For this review, take the finished solid that the model builds, in its own axes (mm). Face numbers are marked on the shaded views. A direction names the side the tool comes from. Round coordinates to 2 decimals unless told otherwise and drop trailing zeros. Order: outer loops, then holes, each group sorted by start corner. A loop starts at its lowest first (then second) coordinate and runs counter-clockwise, first axis right, second up. Notation, with made-up numbers: M 53,56.5 L 76,56.5 A8 cw 76,63.5 Z; hole C -31.5,80.5 d9. An arc over 180 degrees is marked long. Answer in a Markdown table with one row per item. Add a question column.
```python
from build123d import *

# Parameters (mm, degrees)
SKETCH1_R           = 0.499999685
SKETCH1_R_2         = 0.499999936
SKETCH1_R_3         = 3.000000209
SKETCH1_R_4         = 0.750000452
SKETCH1_R_5         = 0.748506913
SKETCH1_R_6         = 1.500187581
BOSS_EXTRUDE1_DEPTH = 4


# Read off the part's stored shape, not the designer's step: Imported1
with BuildPart() as part:
    # Sketch1 → Boss-Extrude1 (new body)
    with BuildSketch(Plane(origin=(0, 0, 0), x_dir=(-1, 0, 0), z_dir=(0, 0, -1))):
        with BuildLine():
            ThreePointArc((-10.3249643, 42.429967422), (-13.429964129, 45.534967549), (-16.534963959, 42.429967422))
            Line((-16.534963959, 42.429967422), (-16.534963959, 22.759328173))
            ThreePointArc((-16.534963959, 22.759328173), (-22.936546798, 10.91939696), (-11.523821193, 3.783997304))
            Line((-11.523821193, 3.783997304), (-11.151510993, 1.898050354))
            ThreePointArc((-11.151510993, 1.898050354), (-7.958448418, 0.172164331), (-6.866399752, 3.633632355))
            Line((-6.866399752, 3.633632355), (-6.907151039, 3.694454964))
            Line((-6.907151039, 3.694454964), (-7.95702579, 5.261426867))
            ThreePointArc((-7.95702579, 5.261426867), (-8.261161621, 6.315782715), (-7.802888126, 7.312853556))
            Line((-7.802888126, 7.312853556), (-7.336401059, 7.778170532))
            ThreePointArc((-7.336401059, 7.778170532), (-6.328947455, 8.250313315), (-5.25191043, 7.971256294))
            Line((-5.25191043, 7.971256294), (-3.681946925, 6.898545358))
            ThreePointArc((-3.681946925, 6.898545358), (-0.18308636, 7.931946592), (-1.898741108, 11.151647221))
            Line((-1.898741108, 11.151647221), (-3.784109013, 11.52325713))
            ThreePointArc((-3.784109013, 11.52325713), (-4.744145314, 12.052872295), (-5.125871494, 13.080708395))
            Line((-5.125871494, 13.080708395), (-5.125914366, 13.778599746))
            Line((-5.125914366, 13.778599746), (-5.125914378, 13.778793202))
            ThreePointArc((-5.125914378, 13.778793202), (-4.744155373, 14.806645767), (-3.783994211, 15.336090171))
            Line((-3.783994211, 15.336090171), (-1.90356186, 15.70732102))
            ThreePointArc((-1.90356186, 15.70732102), (-0.193583134, 18.935202355), (-3.703637126, 19.946521356))
            Line((-3.703637126, 19.946521356), (-5.261386695, 18.902842274))
            ThreePointArc((-5.261386695, 18.902842274), (-6.314757765, 18.59870429), (-7.311417899, 19.055605922))
            Line((-7.311417899, 19.055605922), (-7.805450119, 19.549549653))
            ThreePointArc((-7.805450119, 19.549549653), (-8.262234293, 20.54598288), (-7.957754629, 21.598989571))
            Line((-7.957754629, 21.598989571), (-6.908352, 23.163741071))
            Line((-6.908352, 23.163741071), (-6.866399752, 23.226295558))
            ThreePointArc((-6.866399752, 23.226295558), (-6.774111326, 25.630427698), (-8.842129144, 26.859927922))
            Line((-8.842129144, 26.859927922), (-10.3249643, 26.859927922))
            Line((-10.3249643, 26.859927922), (-10.3249643, 42.429967422))
        make_face()
        with Locations(Location((-15.179963978, 6.929964102, 0), (0, 0, 90))):
            Circle(SKETCH1_R, mode=Mode.SUBTRACT)
        with Locations(Location((-11.679964298, 6.929964382, 0), (0, 0, 90))):
            Circle(SKETCH1_R_2, mode=Mode.SUBTRACT)
        with Locations(Location((-13.42996461, 13.429962781, 0), (0, 0, 90))):
            Circle(SKETCH1_R_3, mode=Mode.SUBTRACT)
        with Locations(Location((-15.179964076, 20.429963954, 0), (0, 0, 90))):
            Circle(SKETCH1_R_4, mode=Mode.SUBTRACT)
        with Locations(Location((-11.681540167, 20.429629577, 0), (0, 0, 90))):
            Circle(SKETCH1_R_5, mode=Mode.SUBTRACT)
        with Locations(Location((-13.429420254, 42.425723706, 0), (0, 0, 90))):
            Circle(SKETCH1_R_6, mode=Mode.SUBTRACT)
    extrude(amount=BOSS_EXTRUDE1_DEPTH)


solid = part.part
```
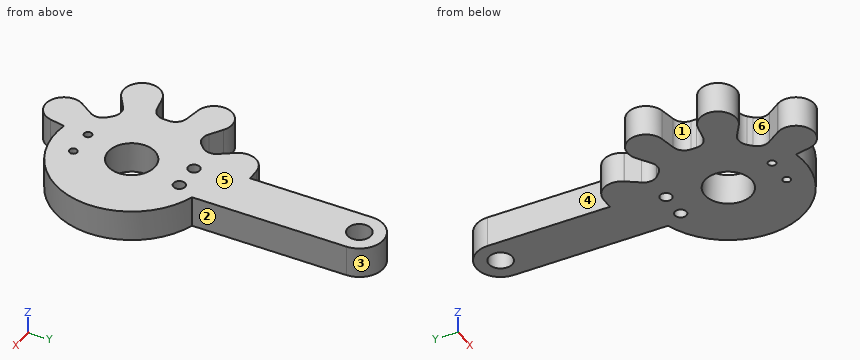
1. Consider section C-C on z = -0.5. State how many separate pieces and enclosed holes the cut face has, plus the area to 3 significant figures.
2. To check wall thickness, follow probe 1 along X at (y, z) = (42.5, -1.4); probe 2 along Y at (x, z) = (13.75, -2.85); probe 3 along X at (y, z) = (41.5, -1.8). State the ranges of each line that lie inside material, in increasing order. Write a range as [from, to].
3. Consider section D-D on y = 40.5. Write out the cut boundary in (x, z), plus the area to 3 significant figures.
4. The part is to be moulded in two halves that separate along X. For the marked faces 4, 5 and 6, say which applies: pulls with the +X half, pulls with the -X half, needs draft (parallel to the pull), parting line crosses it, or undercut.
5. Clearance check with flat-ended pins moving along their axes: pin 1 Ø1 at (x, z) = (11.5, -1.5) entering from +Y; pin 2 Ø2 at (x, z) = (3.5, -1) entering from +Y; pin 3 Ø1.3 at (x, y) = (11.68, 20.43) entering from +Z; pin 4 Ø1.2 at (x, z) = (10, -2.5) entering from +Y. State where each tip first meets the part, or that it passes through.
6. For the marked faces 1, 2 and 3, list the 3-axis set-ups (+Z, -Z, +X, -X, +Y, -Y) from which the entire face can be reached by the end or side of a thin tool; tool diameter is ignored.
7. Consider section B-B on x = 14. Write out the cut boundary in (y, z).
8. Consider section A-A on x = 3. Write out the cut boundary in (y, z), plus the area to 3 significant figures.
Solved:
| question | item | result |
|---|---|---|
| 1 | separate pieces | 1 |
| 1 | enclosed holes | 6 |
| 1 | area | 456 mm^2 |
| 2 | probe 1 | x = [10.33, 11.93], [14.93, 16.53] |
| 2 | probe 2 | y = [3.6, 10.45], [16.41, 40.96], [43.89, 45.52] |
| 2 | probe 3 | x = [10.32, 12.25], [14.61, 16.53] |
| 3 | outline | M 10.32,-4 L 16.53,-4 L 16.53,0 L 10.32,0 Z |
| 3 | area | 24.8 mm^2 |
| 4 | face 4 | pulls with the -X half |
| 4 | face 5 | needs draft |
| 4 | face 6 | undercut |
| 5 | pin 1 | stops at y = 45.19 |
| 5 | pin 2 | stops at y = 20.36 |
| 5 | pin 3 | passes through |
| 5 | pin 4 | stops at y = 43.71 |
| 6 | face 1 | +Z, -Z, -X |
| 6 | face 2 | +Z, -Z, +X, +Y |
| 6 | face 3 | +Z, -Z, +Y |
| 7 | outline | M 3.61,-4 L 10.48,-4 L 10.48,0 L 3.61,0 Z; M 16.38,-4 L 41.04,-4 L 41.04,0 L 16.38,0 Z; M 43.81,-4 L 45.48,-4 L 45.48,0 L 43.81,0 Z |
| 8 | outline | M 6.58,-4 L 11.37,-4 L 11.37,0 L 6.58,0 Z; M 15.49,-4 L 20.28,-4 L 20.28,0 L 15.49,0 Z |
| 8 | area | 38.3 mm^2 |
